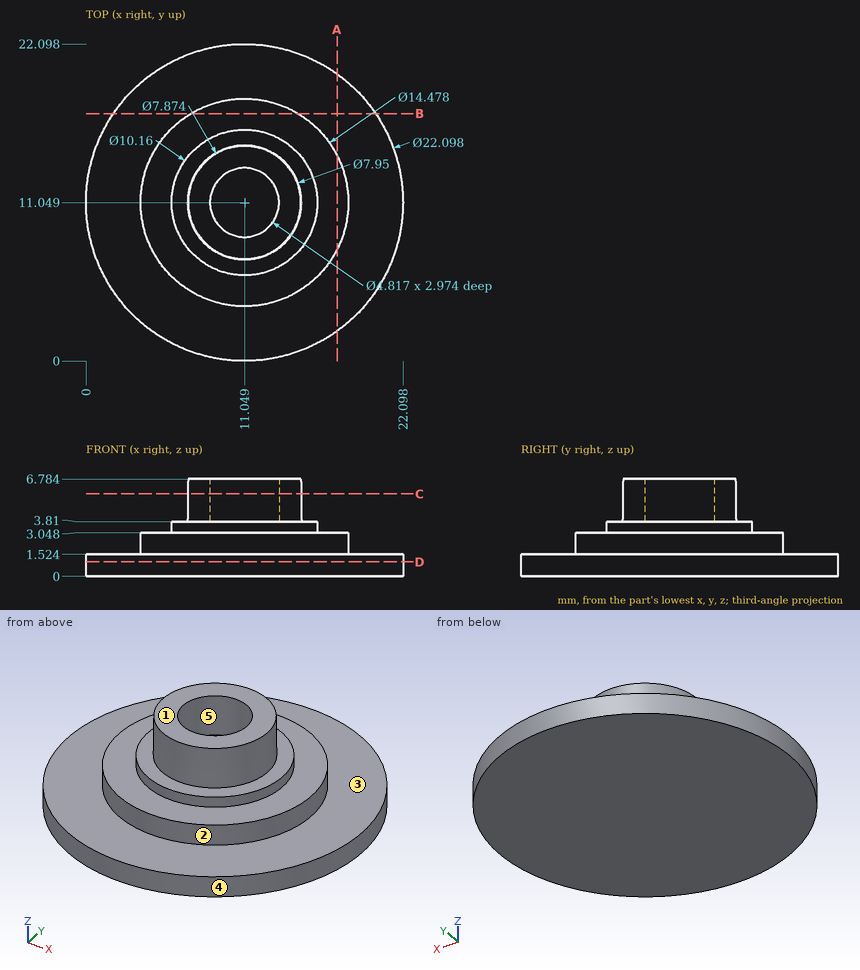
Here's the drawing with two shaded views (mm, measured from the low corner). I have some questions. A direction names the side the tool comes from. Coordinates: 2 decimals unless noted, no trailing zeros. Write each loop counter-clockwise with the first axis right and the second up, starting at its lowest first coordinate (ties: lowest second). Pieces come first, ordered by that corner, then holes. Notation, with made-up numbers: M 17.5,10 L 28.5,10 A15 cw 28.5,37 Z; hole C 2.5,-38.75 d2. An arc over 180 degrees is marked long. Use one line per item in the form item = value.
Q1. If we section it at B-B (y = 17.25): Write out the boundary of the cut face in (x, z).
Model answer:
outline = M 1.9,0 L 20.19,0 L 20.19,1.52 L 14.78,1.52 L 14.78,3.05 L 7.31,3.05 L 7.31,1.52 L 1.9,1.52 Z
Q2. I need wall thicknesses on line 1 along Z through (x, y) = (5, 14.5); line 2 along Z through (x, y) = (2.5, 8.5); line 3 along X through (y, z) = (10, 6) (1 decimal). Which ranges of each line are inside material? Lowest first, please. Write a range as from..to.
Model answer:
line_1 = 0..3.05
line_2 = 0..1.52
line_3 = 7.2..8.9, 13.2..14.9
Q3. If we section it at C-C (z = 5.75): Write out the boundary of the cut face in (x, y).
Model answer:
outline = C 11.05,11.05 d7.9; hole C 11.05,11.05 d4.82
Q4. For P1, Ø4, axis at x = 3.5, z = 1, coming from the -Y side (1 decimal); P2, Ø3, axis at x = 5, y = 5.5, coming from the +Z side, each with a flat end and sliding along its axis, tell me the tip position at first contact or that it passes through.
Model answer:
P1 = 1.5
P2 = 3.05
Q5. If we section it at A-A (x = 17.5): Write out the boundary of the cut face in (y, z) (1 decimal).
Model answer:
outline = M 2.1,0 L 20,0 L 20,1.5 L 14.3,1.5 L 14.3,3 L 7.8,3 L 7.8,1.5 L 2.1,1.5 Z
Q6. For the marked faces 1 and 2, which set-ups out of +Z, -Z, +X, -X, +Y, -Y let a thin tool reach every point of the face, with its end or its side?
Model answer:
face_1 = +Z, +X, -X, +Y, -Y
face_2 = +Z
Q7. We'd pull the mould along Y, two halves only. Please class the marked faces 3, 4 and 5: +Y half, -Y half, draft (parallel to the pull), parting line (faces both ways), or undercut.
Model answer:
face_3 = draft
face_4 = parting line
face_5 = undercut
Q8. If we section it at D-D (z = 1): Write out the boundary of the cut face in (x, y).
Model answer:
outline = C 11.05,11.05 d22.1
